For this review, take the finished solid that the model builds, in its own axes (mm). A direction names the side the tool comes from. Give positions to 0.01 mm unless a question says otherwise; leave off trailing zeros. Write each loop counter-clockwise with the first axis right and the second up, starting at its lowest first coordinate (ties: lowest second). Pieces come first, ordered by that corner, then holes.
1) We need section B-B on x = 0. Give the boundary of the cut face in (y, z), and give its area (3 significant figures).
2) Machinability: for faces 1 (the face through (-25.292, 7.715, -35.718)), 2 (the face through (-0.1, 1.2, -31.5)), 3 (the face through (25, 3, -35)), 4 (the face through (-0.121, -0.986, -37.747)), 5 (the face through (-10.208, 6.521, -31.036)), which of the approach directions +Z, -Z, +X, -X, +Y, -Y give a long, thin tool a straight path to every point of the face, cutting with its end or side? Answer none if there is none.
3) We need section D-D on y = 5.5. Give the boundary of the cut face in (x, z), and give its area (3 significant figures).
4) We need section C-C on z = -33.5. Give the number of separate pieces and of enclosed holes in the cut face, and give its area (3 significant figures).
5) Wall thickness on line 1 along X through (y, z) = (3.5, -33.75); line 2 along X through (y, z) = (3.5, -33); line 3 along Y through (x, z) = (23.5, -36): over which ranges is each line inside the solid? List them lowest first.
6) Draft analysis for pull direction Z (two halves, no side actions). For faces 6 (the face through (6.4, 6.52, -32.42)), 7 (the face through (19.45, 3.55, -31.11)), 8 (the face through (0.352, 7.715, -39.699)), state which applies: pulls with the +Z half, pulls with the -Z half, needs draft (parallel to the pull), parting line crosses it, or undercut.
7) For P1, Ø1.5, axis at x = 2, y = -0.5, coming from the +Z side; P2, Ø3, axis at y = 0, z = -35.5, coming from the -X side; P3, Ø6, axis at x = -18, y = 6.5, coming from the +Z side, all flat-tipped, find the tip position at first contact; note any pin that passes through.
8) We need section A-A on y = 3.25. Give the boundary of the cut face in (x, z).
from build123d import *

# Parameters (mm, degrees)
EXTRUDE_1_DEPTH     = 8
SKETCH_4_R          = 31.5
CUT_EXTRUDE_1_DEPTH = 2.5
SKETCH_5_R          = 1.5
CUT_EXTRUDE_2_DEPTH = 51.635955605
SKETCH_6_R          = 3
CUT_EXTRUDE_3_DEPTH = 3
SKETCH_7_R          = 2.75
EXTRUDE_2_DEPTH     = 2
FILLET_1_R          = 15
FILLET_2_R          = 2
FILLET_3_R          = 1


with BuildPart() as part:
    # 草图3 → 凸台-拉伸1 (new body)
    with BuildSketch(Plane(origin=(0, 0, 0), x_dir=(1, 0, 0), z_dir=(0, 1, 0))):
        Polygon((-20, 30), (20, 30), (30, 40), (-30, 40), align=None)
    extrude(amount=EXTRUDE_1_DEPTH)

    # 草图4 → 切除-拉伸1 (cut)
    with BuildSketch(Plane.XZ):
        Circle(SKETCH_4_R)
    extrude(amount=-CUT_EXTRUDE_1_DEPTH, mode=Mode.SUBTRACT)

    # 草图5 → 切除-拉伸2 (cut, through all)
    with BuildSketch(Plane(origin=(0, 8, 0), x_dir=(1, 0, 0), z_dir=(0, 1, 0))):
        with Locations(Location((-9.058666579, 33.80740392, 0), (0, 0, 270))):
            Circle(SKETCH_5_R)
        with Locations(Location((9.058666579, 33.80740392, 0), (0, 0, 90))):
            Circle(SKETCH_5_R)
    extrude(amount=-CUT_EXTRUDE_2_DEPTH, mode=Mode.SUBTRACT)

    # 草图6 → 切除-拉伸3 (cut)
    with BuildSketch(Plane(origin=(0, 8, 0), x_dir=(1, 0, 0), z_dir=(0, 1, 0))):
        with Locations(Location((-9.058666579, 33.80740392, 0), (0, 0, 270))):
            Circle(SKETCH_6_R)
        with Locations(Location((9.058666579, 33.80740392, 0), (0, 0, 270))):
            Circle(SKETCH_6_R)
    extrude(amount=-CUT_EXTRUDE_3_DEPTH, mode=Mode.SUBTRACT)

    # 草图7 → 凸台-拉伸2 (add)
    with BuildSketch(Plane.XZ):
        with Locations(Location((0, -35, 0), (0, 0, 90))):
            Circle(SKETCH_7_R)
    extrude(amount=EXTRUDE_2_DEPTH)

    # 圆角1
    fillet_1_edges = [part.edges().sort_by_distance(p)[0] for p in [
        (20, 4, -30),
        (-20, 4, -30),
    ]]
    fillet(fillet_1_edges, radius=FILLET_1_R)

    # 圆角2
    fillet_2_edges = [part.edges().sort_by_distance(p)[0] for p in [
        (-30, 4, -40),
        (30, 4, -40),
    ]]
    fillet(fillet_2_edges, radius=FILLET_2_R)

    # 圆角3
    # the kernel refuses this fillet: 1 mm, written as the material it takes off along each edge
    with BuildSketch(Plane(origin=(24.393398282, 8, -34.393398282), x_dir=(0, -1, 0), z_dir=(0.7071067811865472, 0, -0.7071067811865478)), Plane(origin=(-26.585786438, 8, -36.585786438), x_dir=(0, -1, 0), z_dir=(0.7071067811865472, 0, 0.7071067811865478))) as fillet_3_piece_1:
        with BuildLine():
            CenterArc((FILLET_3_R, FILLET_3_R), FILLET_3_R, 180, 90)
            Line((0, FILLET_3_R), (0, 0))
            Line((0, 0), (FILLET_3_R, 0))
        make_face()
    extrude(amount=3.100505063, mode=Mode.SUBTRACT)
    with BuildSketch(Plane(origin=(-13.786796564, 8, -30), x_dir=(0, -1, 0), z_dir=(1, 0, 0))) as fillet_3_piece_2:
        with BuildLine():
            CenterArc((FILLET_3_R, FILLET_3_R), FILLET_3_R, 180, 90)
            Line((0, FILLET_3_R), (0, 0))
            Line((0, 0), (FILLET_3_R, 0))
        make_face()
    extrude(amount=27.573593129, mode=Mode.SUBTRACT)
    with BuildSketch(Plane(origin=(-13.786796564, 8, -45), x_dir=(0, 0, 1), z_dir=(1, 0, 0))) as fillet_3_piece_3:
        with BuildLine():
            CenterArc((15 - FILLET_3_R, FILLET_3_R), FILLET_3_R, 270, 90)
            Line((15 - FILLET_3_R, 0), (15, 0))
            Line((15, 0), (15, FILLET_3_R))
        make_face()
    revolve(axis=Axis((-13.786796564, 8, -45), (0, -1, 0)), revolution_arc=45, mode=Mode.SUBTRACT)
    with BuildSketch(Plane(origin=(13.786796564, 8, -45), x_dir=(0, 0, 1), z_dir=(-1, 0, 0))) as fillet_3_piece_4:
        with BuildLine():
            CenterArc((15 - FILLET_3_R, -FILLET_3_R), FILLET_3_R, 0, 90)
            Line((15 - FILLET_3_R, 0), (15, 0))
            Line((15, 0), (15, -FILLET_3_R))
        make_face()
    revolve(axis=Axis((13.786796564, 8, -45), (0, 1, 0)), revolution_arc=45, mode=Mode.SUBTRACT)
    with BuildSketch(Plane(origin=(25.171572875, 8, -40), x_dir=(0, -1, 0), z_dir=(-1, 0, 0))) as fillet_3_piece_5:
        with BuildLine():
            CenterArc((FILLET_3_R, FILLET_3_R), FILLET_3_R, 180, 90)
            Line((0, FILLET_3_R), (0, 0))
            Line((0, 0), (FILLET_3_R, 0))
        make_face()
    extrude(amount=50.343145751, mode=Mode.SUBTRACT)
    with BuildSketch(Plane(origin=(-25.171572875, 8, -38), x_dir=(-0.7071067811865458, 0, 0.7071067811865493), z_dir=(0.7071067811865493, 0, 0.7071067811865458))) as fillet_3_piece_6:
        with BuildLine():
            CenterArc((2 - FILLET_3_R, FILLET_3_R), FILLET_3_R, 270, 90)
            Line((2 - FILLET_3_R, 0), (2, 0))
            Line((2, 0), (2, FILLET_3_R))
        make_face()
    revolve(axis=Axis((-25.171572875, 8, -38), (0, -1, 0)), revolution_arc=135, mode=Mode.SUBTRACT)
    with BuildSketch(Plane(origin=(25.171572875, 8, -38), x_dir=(0, 0, -1), z_dir=(-1, 0, 0))) as fillet_3_piece_7:
        with BuildLine():
            CenterArc((2 - FILLET_3_R, FILLET_3_R), FILLET_3_R, 270, 90)
            Line((2 - FILLET_3_R, 0), (2, 0))
            Line((2, 0), (2, FILLET_3_R))
        make_face()
    revolve(axis=Axis((25.171572875, 8, -38), (0, -1, 0)), revolution_arc=135, mode=Mode.SUBTRACT)


solid = part.part
Results list:
1. outline: (-2, -37.75) - (0, -37.75) - (0, -40) - (7, -40) arc R1 ccw to (8, -39) - (8, -31) arc R1 ccw to (7, -30) - (2.5, -30) - (2.5, -31.5) - (0, -31.5) - (0, -32.25) - (-2, -32.25) - close
1. area: 86.8 mm2
2. face 1: +Z, -X, +Y
2. face 2: +Z, -Y
2. face 3: +Z, +X, +Y, -Y
2. face 4: -Y
2. face 5: +Y
3. outline: (-26.59, -36.59) arc R2 ccw to (-25.17, -40) - (25.17, -40) arc R2 ccw to (26.59, -36.59) - (24.39, -34.39) arc R15 ccw to (13.79, -30) - (-13.79, -30) arc R15 ccw to (-24.39, -34.39) - close; hole circle Ø6 at (-9.06, -33.81); hole circle Ø6 at (9.06, -33.81)
3. area: 424 mm2
4. separate pieces: 3
4. enclosed holes: 0
4. area: 318 mm2
5. line 1: x = -23.71 to -10.56, -7.56 to 7.56, 10.56 to 23.71
5. line 2: x = -22.79 to -10.32, -7.79 to 7.79, 10.32 to 22.79
5. line 3: y = 0 to 8
6. face 6: undercut
6. face 7: pulls with the +Z half
6. face 8: pulls with the -Z half
7. P1: stops at z = -31.4
7. P2: stops at x = -26.9
7. P3: stops at z = -30.05
8. outline: (-26.59, -36.59) arc R2 ccw to (-25.17, -40) - (25.17, -40) arc R2 ccw to (26.59, -36.59) - (24.39, -34.39) arc R15 ccw to (13.79, -30) - (-13.79, -30) arc R15 ccw to (-24.39, -34.39) - close; hole circle Ø3 at (-9.06, -33.81); hole circle Ø3 at (9.06, -33.81)
